Autodesk Inventor part; units mm, degrees
ref_plane "Work Plane1" through (0, 0, 43.18) normal (0, 0, 1) x (1, 0, 0)
ref_plane "Work Plane8" through (-25.6243, 32.385, 63.5) normal (0, -1, 0) x (1, 0, 0)
ref_plane "Work Plane9" through (0, 12.065, 31.75) normal (0, 1, 0) x (1, 0, 0)
sketch "Sketch1" plane through (0, 0, 0) normal (0, 0, 1) x (1, 0, 0)
  circle A0 centre (0, 0) radius 13.97
  circle A1 centre (0, 0) radius 10.795
  dimension "d0" = 27.94
  dimension "d2" = 21.59
extrude "Extrusion1" add sketch "Sketch1" along normal blind 63.5
ref_plane "Work Plane1" through (0, 0, 43.18) normal (0, 0, 1) x (1, 0, 0)
sketch "Sketch2" plane through (0, 0, 43.18) normal (0, 0, 1) x (1, 0, 0)
  circle A0 centre (0, 0) radius 10.414
  circle A1 centre (0, 0) radius 10.795
  dimension "d6" = 20.828
  dimension "d9" = 21.59
extrude "Extrusion2" add sketch "Sketch2" against normal blind 28.829
sketch "Sketch3" plane through (0, 0, 63.5) normal (0, 0, 1) x (1, 0, 0)
  circle A0 centre (0, 0) radius 10.795
  circle A1 centre (0, 0) radius 13.97
  line L0 (-25.6243, 13.97) -> (27.2368, 13.97)
ref_plane "Work Plane8" through (-25.6243, 32.385, 63.5) normal (0, -1, 0) x (1, 0, 0)
ref_plane "Work Plane7" through (-25.6243, 13.97, 63.5) normal (0, -1, 0) x (1, 0, 0)
sketch "Sketch10" plane through (0, 0, 0) normal (0, 0, -1) x (-1, 0, 0)
  circle A0 centre (0, 0) radius 10.795
extrude "Extrusion8" cut sketch "Sketch10" against normal blind 20.32
sketch "Sketch11" plane through (-25.6243, 32.385, 63.5) normal (0, -1, 0) x (1, 0, 0)
  circle A0 centre (25.6243, -31.75) radius 13.97
  circle A1 centre (25.6243, -31.75) radius 10.795
  point P0 (25.6243, -63.5)
  dimension "d45" = 31.75
  dimension "d46" = 27.94
  dimension "d47" = 21.59
extrude "Extrusion9" add sketch "Sketch11" along normal blind 32.385
sketch "Sketch12" plane through (0, 0, 43.18) normal (0, 0, 1) x (1, 0, 0)
  arc A0 (-8.0322, 6.6284) -> (8.0322, 6.6284) centre (0, 0) ccw
  circle A1 centre (0, 0) radius 10.414
extrude "Extrusion10" cut sketch "Sketch12" against normal blind 76.2
sketch "Sketch13" plane through (0, 32.385, 31.75) normal (0, 1, 0) x (1, 0, 0)
  circle A0 centre (0, 0) radius 10.795
  point P0 (0, 31.75)
extrude "Extrusion11" cut sketch "Sketch13" against normal blind 32.385
ref_plane "Work Plane9" through (0, 12.065, 31.75) normal (0, 1, 0) x (1, 0, 0)
sketch "Sketch14" plane through (0, 12.065, 31.75) normal (0, 1, 0) x (1, 0, 0)
  circle A0 centre (0, 0) radius 10.795
  circle A1 centre (0, 0) radius 10.414
  point P0 (0, 31.75)
  dimension "d55" = 21.59
  dimension "d57" = 20.828
extrude "Extrusion12" add sketch "Sketch14" against normal blind 12.7
extrude "Extrusion13" cut sketch "Sketch2" along normal mid plane 76.2 contours A0
sketch "Sketch15" plane through (0, 0, 63.5) normal (0, 0, 1) x (1, 0, 0)
  circle A0 centre (0, 0) radius 10.795
extrude "Extrusion14" cut sketch "Sketch15" against normal blind 20.32
sketch "Sketch16" plane through (0, 0, 0) normal (0, 0, -1) x (-1, 0, 0)
  circle A0 centre (0, 0) radius 10.795
extrude "Extrusion15" cut sketch "Sketch16" against normal blind 20.32
ref_plane "Work Plane10" through (0, 0.635, 31.75) normal (0, 1, 0) x (1, 0, 0)
sketch "Sketch17" plane through (0, 0.635, 31.75) normal (0, 1, 0) x (1, 0, 0)
  line L0 (-45.1678, 43.2051) -> (58.2697, 43.2051)
  line L1 (58.2697, 43.2051) -> (58.2697, -50.7572)
  line L2 (58.2697, -50.7572) -> (-45.1678, -50.7572)
  line L3 (-45.1678, -50.7572) -> (-45.1678, 43.2051)
  point P0 (0, 31.75)
extrude "Extrusion16" cut sketch "Sketch17" against normal blind 25.4
sketch "Sketch18" plane through (0, 0, 63.5) normal (0, 0, 1) x (1, 0, 0)
  line L0 (-13.9556, 0.635) -> (-10.7763, 0.635)
  arc A0 (10.7763, 0.635) -> (-10.7763, 0.635) centre (0, 0) ccw
  line L1 (10.7763, 0.635) -> (13.9556, 0.635)
  arc A1 (13.9556, 0.635) -> (-13.9556, 0.635) centre (0, 0) ccw
extrude "Extrusion17" cut sketch "Sketch18" against normal blind 12.7
sketch "Sketch19" plane through (0, 0, 0) normal (0, 0, -1) x (-1, 0, 0)
  line L0 (10.7763, 0.635) -> (13.9556, 0.635)
  arc A0 (13.9556, 0.635) -> (-13.9556, 0.635) centre (0, 0) ccw
  line L1 (-13.9556, 0.635) -> (-10.7763, 0.635)
  arc A1 (10.7763, 0.635) -> (-10.7763, 0.635) centre (0, 0) ccw
extrude "Extrusion18" cut sketch "Sketch19" against normal blind 12.7
ref_plane "Work Plane11" through (-10.7763, 0.635, 0) normal (-1, 0, 0) x (0, 0, -1)
sketch "Sketch20" plane through (-10.7763, 0.635, 0) normal (-1, 0, 0) x (0, 0, -1)
  arc A0 (-47.625, -3.175) -> (-44.45, -3.175) centre (-46.0375, -3.175) ccw
  line L0 (-44.45, -3.175) -> (-44.45, 0)
  line L1 (-44.45, 0) -> (-47.625, 0)
  line L2 (-47.625, 0) -> (-47.625, -3.175)
  point P0 (0, 0.635)
  point P1 (-50.8, 0)
  point P2 (-46.0375, 0)
  dimension "d74" = 0.635
  dimension "d75" = 50.8
  dimension "d76" = 3.175
  dimension "d77" = 3.175
  dimension "d78" = 1.5875
  dimension "d79" = 3.175
extrude "Extrusion19" cut sketch "Sketch20" along normal mid plane 50.8
properties part number "0.5 Frame Mount" material "PVC-Piping"
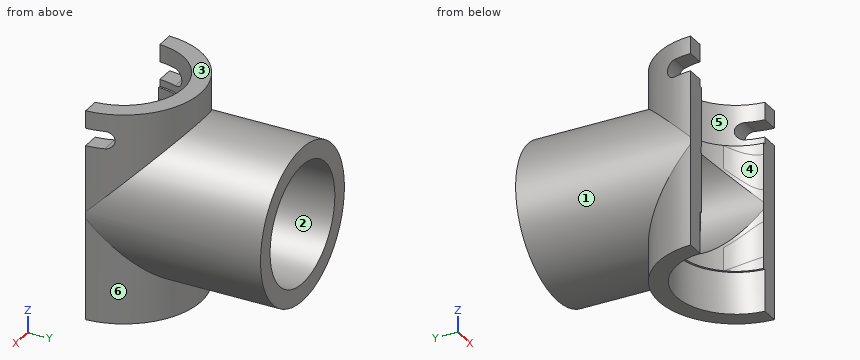
Source: CAD feature listing. Evaluate the final solid. Frame: model axes, mm. Face numbers are marked on the shaded views. A direction names the side the tool comes from. Round coordinates to 2 decimals unless told otherwise and drop trailing zeros. Loops run counter-clockwise (first coordinate to the right, second up) from the corner with the lowest first, then second, coordinate; pieces in that order, holes last.
Q1. First-contact query: P1, Ø8, axis at x = 3, y = 4, coming from the +Z side; P2, Ø3, axis at y = 22.5, z = 39, coming from the +X side; P3, Ø6, axis at y = 25, z = 40.5, coming from the -X side; P4, Ø5, axis at x = -11, y = 11.5, coming from the -Z side. Flat tips, straight axial feed; report the tip coordinate or a pass-through.
Q2. Section A-A, the plane x = 0. Return loops of the section in (y, z) (3 decimals), plus the area to 3 significant figures.
Q3. Section C-C, the plane y = 3. State how many separate pieces and enclosed holes the cut face has, plus the area to 3 significant figures.
Q4. Ray query, line 1 (Z direction, x = 0, y = 20.25) (3 decimals); line 2 (X direction, y = 6, z = 31); line 3 (X direction, y = 24, z = 31). Return the intervals inside material, ascending.
Q5. Section D-D, the plane z = 16.5. Return loops of the section in (x, y) (3 decimals), plus the area to 3 significant figures.
Q6. Access query for the marked faces 4, 5 and 6. Directions: +Z, -Z, +X, -X, +Y, -Y. A direction counts if a zero-diameter tool reaches every point of the face in a straight line with its end or side. Return the directions, or none.
Q7. Section B-B, the plane z = 31.75. Return loops of the section in (x, y) (3 decimals), plus the area to 3 significant figures.
Q8. Mould query, pull axis Z, two halves, no side actions, for the marked faces 1, 2 and 3. Classes: pulls with the +Z half, pulls with the -Z half, needs draft (parallel to the pull), parting line crosses it, or undercut.
Solutions:
1. P1: passes through
1. P2: stops at x = 12.73
1. P3: stops at x = -12.73
1. P4: stops at z = 12.7
2. outline: (10.414, 20.32) - (10.795, 20.32) - (10.795, 12.7) - (13.97, 12.7) - (13.97, 17.78) - (32.385, 17.78) - (32.385, 20.955) - (12.065, 20.955) - (12.065, 21.336) - (10.414, 21.336) - close; (10.414, 42.164) - (12.065, 42.164) - (12.065, 42.545) - (32.385, 42.545) - (32.385, 45.72) - (13.97, 45.72) - (13.97, 50.8) - (10.795, 50.8) - (10.795, 43.18) - (10.414, 43.18) - close
2. area: 171 mm2
3. separate pieces: 4
3. enclosed holes: 0
3. area: 246 mm2
4. line 1: z = 17.78 to 20.955, 42.545 to 45.72
4. line 2: x = -13.95 to -10.39, 10.39 to 13.95
4. line 3: x = -13.95 to -10.77, 10.77 to 13.95
5. outline: (-13.956, 0.635) - (-10.776, 0.635) arc R10.795 cw to (10.776, 0.635) - (13.956, 0.635) arc R13.97 ccw to start
5. area: 119 mm2
6. face 4: +Z, -Z, -Y
6. face 5: +Z, -Y
6. face 6: -Z, +Y
7. outline: (-13.97, 0.635) - (-10.414, 0.635) - (-10.414, 12.065) - (-10.795, 12.065) - (-10.795, 32.385) - (-13.97, 32.385) - close; (10.414, 0.635) - (13.97, 0.635) - (13.97, 32.385) - (10.795, 32.385) - (10.795, 12.065) - (10.414, 12.065) - close
7. area: 210 mm2
8. face 1: parting line crosses it
8. face 2: undercut
8. face 3: pulls with the +Z half
